from build123d import *

# Parameters (mm, degrees)
F1_DEPTH = 3
F2_R     = 0.5
F3_DEPTH = 3


# Not quite as in the source:
# - a feature names something its author has since deleted; it is built from what else it names


with BuildPart() as f1:
    # F0 (on Front) → F1 (new body)
    with BuildSketch(Plane.XZ):
        with BuildLine():
            Line((0, 10), (0, 0))
            Line((0, 0), (33, 0))
            Line((33, 0), (33, 3))
            Line((33, 3), (73, 3))
            Line((73, 3), (73, 0))
            Line((73, 0), (143, 0))
            Line((143, 0), (143, 3))
            Line((143, 3), (183, 3))
            Line((183, 3), (183, 0))
            Line((183, 0), (216, 0))
            Line((216, 0), (216, 70))
            Line((216, 70), (213, 70))
            Line((213, 70), (213, 125))
            Line((213, 125), (216, 125))
            Line((216, 125), (216, 185))
            Line((216, 185), (213, 185))
            Line((213, 185), (213, 240))
            Line((213, 240), (216, 240))
            Line((216, 240), (216, 300))
            Line((216, 300), (211, 300))
            Line((211, 300), (211, 297))
            Line((211, 297), (181, 297))
            Line((181, 297), (181, 300))
            Line((181, 300), (176, 300))
            Line((176, 300), (174.706427271, 297))
            Line((174.706427271, 297), (161.7706999809, 267))
            Line((161.7706999809, 267), (152.9198643438, 246.4735105991))
            Line((152.9198643438, 246.4735105991), (108.8058184443, 144.1660525563))
            add(Edge.make_bspline(
                [(5.2380922861, 115.1536645525), (67.1986155562, 116.9837427001), (97.7651412543, 118.5609738259), (108.8058184443, 144.1660525563)],
                knots=[3.0455141627, 3.0455141627, 3.0455141627, 3.0455141627, 112.6470805172, 112.6470805172, 112.6470805172, 112.6470805172], degree=3))
            ThreePointArc((5.2380922861, 115.1536645525), (1.636924279, 112.8542013763), (0, 108.9075039192))
            Line((0, 108.9075039192), (0, 107.6488941908))
            Line((0, 107.6488941908), (0, 95))
            Line((0, 95), (3, 95))
            Line((3, 95), (3, 60))
            Line((3, 60), (0, 60))
            Line((0, 60), (0, 45))
            Line((0, 45), (3, 45))
            Line((3, 45), (3, 10))
            Line((3, 10), (0, 10))
        make_face()
        Polygon((54.8936169141, 111.7298124622), (54.5449186418, 114.7094784694), (104.2060187631, 120.5211163403), (104.5547170354, 117.541450333), align=None, mode=Mode.SUBTRACT)
        Polygon((129.52643753, 177.6246576271), (151.3037139596, 228.1296101695), (154.0585295529, 226.9417587279), (132.2812531233, 176.4368061855), align=None, mode=Mode.SUBTRACT)
        Polygon((146, 267), (161.7706999809, 267), (174.706427271, 297), (146, 297), (146, 292), (149, 292), (149, 272), (146, 272), align=None)
        Polygon((146, 297), (174.706427271, 297), (176, 300), (146, 300), align=None)
        with BuildLine():
            add(Edge.make_bspline(
                [(146, 267), (156.1105200986, 267), (157.3542433109, 256.7575376221), (152.9198643438, 246.4735105991)],
                knots=[0, 0, 0, 0, 21.6615163288, 21.6615163288, 21.6615163288, 21.6615163288], degree=3))
            Line((152.9198643438, 246.4735105991), (161.7706999809, 267))
            Line((161.7706999809, 267), (146, 267))
        make_face()
    extrude(amount=F1_DEPTH)

    # F2 (on face) → F3 (cut, through all)
    with BuildSketch(Plane.XZ.offset(3)):
        with Locations((41.5442730218, 42.1421974897)):
            Circle(F2_R)
        with Locations((47.2275130451, 42.1421974897)):
            Circle(F2_R)
        with Locations((53.483594209, 42.1421974897)):
            Circle(F2_R)
        with Locations((59.3261942267, 42.1421974897)):
            Circle(F2_R)
        with Locations((45.5629305814, 46.1608550493)):
            Circle(F2_R)
        with Locations((41.5442730218, 47.825437513)):
            Circle(F2_R)
        with Locations((37.5256154622, 46.1608550493)):
            Circle(F2_R)
        with Locations((35.8610329985, 42.1421974897)):
            Circle(F2_R)
        with Locations((37.5256154622, 38.1235399302)):
            Circle(F2_R)
        with Locations((41.5442730218, 36.4589574665)):
            Circle(F2_R)
        with Locations((45.5629305814, 38.1235399302)):
            Circle(F2_R)
        with Locations((52.4513856597, 46.99835691)):
            Circle(F2_R)
        with Locations((49.5332382473, 51.0148422497)):
            Circle(F2_R)
        with Locations((45.2337261699, 53.4971667049)):
            Circle(F2_R)
        with Locations((40.2962741256, 54.0161138262)):
            Circle(F2_R)
        with Locations((35.5746124282, 52.4819529418)):
            Circle(F2_R)
        with Locations((31.8851592801, 49.1599544059)):
            Circle(F2_R)
        with Locations((29.8658546482, 44.624521945)):
            Circle(F2_R)
        with Locations((29.8658546482, 39.6598730345)):
            Circle(F2_R)
        with Locations((31.8851592801, 35.1244405735)):
            Circle(F2_R)
        with Locations((35.5746124282, 31.8024420377)):
            Circle(F2_R)
        with Locations((40.2962741256, 30.2682811533)):
            Circle(F2_R)
        with Locations((45.2337261699, 30.7872282745)):
            Circle(F2_R)
        with Locations((49.5332382473, 33.2695527298)):
            Circle(F2_R)
        with Locations((52.4513856597, 37.2860380695)):
            Circle(F2_R)
        with Locations((58.7675424734, 46.5643814678)):
            Circle(F2_R)
        with Locations((57.1266893577, 50.7087033628)):
            Circle(F2_R)
        with Locations((54.5067357155, 54.3147601884)):
            Circle(F2_R)
        with Locations((51.0723028696, 57.1559701322)):
            Circle(F2_R)
        with Locations((47.0391888668, 59.053809524)):
            Circle(F2_R)
        with Locations((42.6608090925, 59.8890301351)):
            Circle(F2_R)
        with Locations((38.2122732505, 59.6091519828)):
            Circle(F2_R)
        with Locations((33.9730992085, 58.2317608408)):
            Circle(F2_R)
        with Locations((30.2096498619, 55.8434032602)):
            Circle(F2_R)
        with Locations((27.1583965743, 52.5941485314)):
            Circle(F2_R)
        with Locations((25.0110608115, 48.6881592792)):
            Circle(F2_R)
        with Locations((23.9025675767, 44.3708631733)):
            Circle(F2_R)
        with Locations((23.9025675767, 39.9135318061)):
            Circle(F2_R)
        with Locations((25.0110608115, 35.5962357003)):
            Circle(F2_R)
        with Locations((27.1583965743, 31.690246448)):
            Circle(F2_R)
        with Locations((30.2096498619, 28.4409917193)):
            Circle(F2_R)
        with Locations((33.9730992085, 26.0526341387)):
            Circle(F2_R)
        with Locations((38.2122732505, 24.6752429966)):
            Circle(F2_R)
        with Locations((42.6608090925, 24.3953648444)):
            Circle(F2_R)
        with Locations((47.0391888668, 25.2305854555)):
            Circle(F2_R)
        with Locations((51.0723028696, 27.1284248473)):
            Circle(F2_R)
        with Locations((54.5067357155, 29.969634791)):
            Circle(F2_R)
        with Locations((57.1266893577, 33.5756916167)):
            Circle(F2_R)
        with Locations((58.7675424734, 37.7200135117)):
            Circle(F2_R)
    extrude(amount=-F3_DEPTH, mode=Mode.SUBTRACT)


solid = f1.part
Input: part model. Units: mm. Frame: model coordinates. A direction names the side the tool comes from. Coordinates: 2 decimals unless noted, no trailing zeros. Loops run counter-clockwise (first coordinate to the right, second up) from the corner with the lowest first, then second, coordinate; pieces in that order, holes last. Notation, with made-up numbers: (69, -7) -> (102, -7) arc R24 ccw to (102, 18) -> close; hole circle Ø3 at (1, 89.5). An arc over 180 degrees is marked (long way). Write item = value, one per line. Start each with the question number.
Item 1: Cut plane B-B, the plane y = -1.75. Count the separate pieces of the cut face and the enclosed holes in it, plus the area to 3 significant figures.
Item 2: Reachability of faces 4 (the face through (130, 0, 119)), 5 (the face through (80.072, -1.479, 114.676)) from +Z, -Z, +X, -X, +Y, -Y: full face, straight path, thin tool, end or side. Return the list, or none.
Item 3: Mould query, pull axis Z, two halves, no side actions, for faces 1 (the face through (130, -3, 119)), 2 (the face through (143.32, -1.48, 202.04)), 3 (the face through (140.26, -1.48, 202.52)). Classes: pulls with the +Z half, pulls with the -Z half, needs draft (parallel to the pull), parting line crosses it, or undercut.
Item 4: Cut plane C-C, the plane x = 116.5. Return loops of the section in (y, z), plus the area to 3 significant figures.
Item 5: First-contact query: P1, Ø0.9, axis at y = -1.5, z = 280.5, coming from the -X side; P2, Ø1.5, axis at y = -2, z = 33.5, coming from the -X side; P3, Ø1.5, axis at x = 172.5, y = -1, coming from the -Z side. Flat tips, straight axial feed; report the tip coordinate or a pass-through.
Item 6: Material intervals for line 1 (X direction, y = -0.5, z = 32); line 2 (Z direction, x = 29.5, y = -1); line 3 (Z direction, x = 190, y = -1.55), sorted ascending.
Item 7: Cut plane A-A, the plane z = 218.5. Return loops of the section in (x, y), plus the area to 3 significant figures.
Ans:
q1.separate_pieces = 1
q1.enclosed_holes = 51
q1.area = 39,500 mm²
q2.face_4 = +Z, -Z, +X, -X, +Y
q2.face_5 = +Y, -Y
q3.face_1 = needs draft
q3.face_2 = undercut
q3.face_3 = undercut
q4.outline = (-3, 0) -> (0, 0) -> (0, 162.01) -> (-3, 162.01) -> close
q4.area = 486 mm²
q5.P1 = 149
q5.P2 = 3
q5.P3 = 3
q6.line_1 = 3 to 26.77, 27.55 to 35.12, 36.03 to 216
q6.line_2 = 0 to 39.32, 40 to 44.28, 44.97 to 115.98
q6.line_3 = 0 to 297
q7.outline = (140.86, -3) -> (147.15, -3) -> (147.15, 0) -> (140.86, 0) -> close; (150.42, -3) -> (213, -3) -> (213, 0) -> (150.42, 0) -> close
q7.area = 207 mm²
